```python
from build123d import *

# Parameters (mm, degrees)
F1_DEPTH = 749


with BuildPart() as f1:
    # F0 (on Front) → F1 (new body)
    with BuildSketch(Plane.XZ):
        with BuildLine():
            ThreePointArc((45, 39), (43.242641, 43.242641), (39, 45))
            Line((39, 45), (-39, 45))
            ThreePointArc((-39, 45), (-43.242641, 43.242641), (-45, 39))
            Line((-45, 39), (-45, -39))
            ThreePointArc((-45, -39), (-43.242641, -43.242641), (-39, -45))
            Line((-39, -45), (39, -45))
            ThreePointArc((39, -45), (43.242641, -43.242641), (45, -39))
            Line((45, -39), (45, 39))
        make_face()
        with BuildLine():
            ThreePointArc((-41, 39), (-40.414214, 40.414214), (-39, 41))
            Line((-39, 41), (39, 41))
            ThreePointArc((39, 41), (40.414214, 40.414214), (41, 39))
            Line((41, 39), (41, -39))
            ThreePointArc((41, -39), (40.414214, -40.414214), (39, -41))
            Line((39, -41), (-39, -41))
            ThreePointArc((-39, -41), (-40.414214, -40.414214), (-41, -39))
            Line((-41, -39), (-41, 39))
        make_face(mode=Mode.SUBTRACT)
    extrude(amount=-F1_DEPTH)


solid = f1.part
```
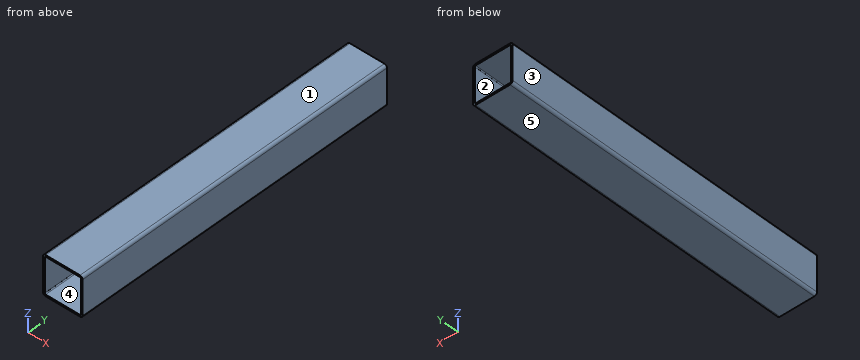
The model under review builds one solid part; all positions refer to its coordinate system, in mm. Face numbers are marked on the shaded views. A direction names the side the tool comes from. Give positions to 0.01 mm unless a question says otherwise; leave off trailing zeros. Write each loop counter-clockwise with the first axis right and the second up, starting at its lowest first coordinate (ties: lowest second). Pieces come first, ordered by that corner, then holes.
(1) Consider section B-B, the plane y = 376. Give the boundary of the cut face in (x, z).
(2) Tool access review of the marked faces 4 and 5: name each direction out of +Z, -Z, +X, -X, +Y, -Y from which nothing blocks a thin tool from reaching the whole face with its end or side.
(3) Consider section A-A, the plane x = 18. Give the boundary of the cut face in (y, z), and give its area (3 significant figures).
(4) The part is to be moulded in two halves that separate along X. For the marked faces 1, 2 and 3, say which applies: released by +X, released by -X, zero draft, split by the parting line, or undercut.
(5) To check wall thickness, follow L1, parallel to Z at x = -28, y = 438; L2, parallel to Z at x = -40, y = 616. State the ranges of each line that lie inside material, in increasing order.
(6) Consider section C-C, the plane z = -23. Give the boundary of the cut face in (x, y).
Returned:
1. outline: (-45, -39) arc R6 ccw to (-39, -45) - (39, -45) arc R6 ccw to (45, -39) - (45, 39) arc R6 ccw to (39, 45) - (-39, 45) arc R6 ccw to (-45, 39) - close; hole (-41, -39) arc R2 ccw to (-39, -41) - (39, -41) arc R2 ccw to (41, -39) - (41, 39) arc R2 ccw to (39, 41) - (-39, 41) arc R2 ccw to (-41, 39) - close
2. face 4: +Y, -Y
2. face 5: -Z, +X, -X, +Y, -Y
3. outline: (0, -45) - (749, -45) - (749, -41) - (0, -41) - close; (0, 41) - (749, 41) - (749, 45) - (0, 45) - close
3. area: 5,990 mm2
4. face 1: zero draft
4. face 2: undercut
4. face 3: released by -X
5. L1: z = -45 to -41, 41 to 45
5. L2: z = -44.92 to -40.73, 40.73 to 44.92
6. outline: (-45, 0) - (-41, 0) - (-41, 749) - (-45, 749) - close; (41, 0) - (45, 0) - (45, 749) - (41, 749) - close
